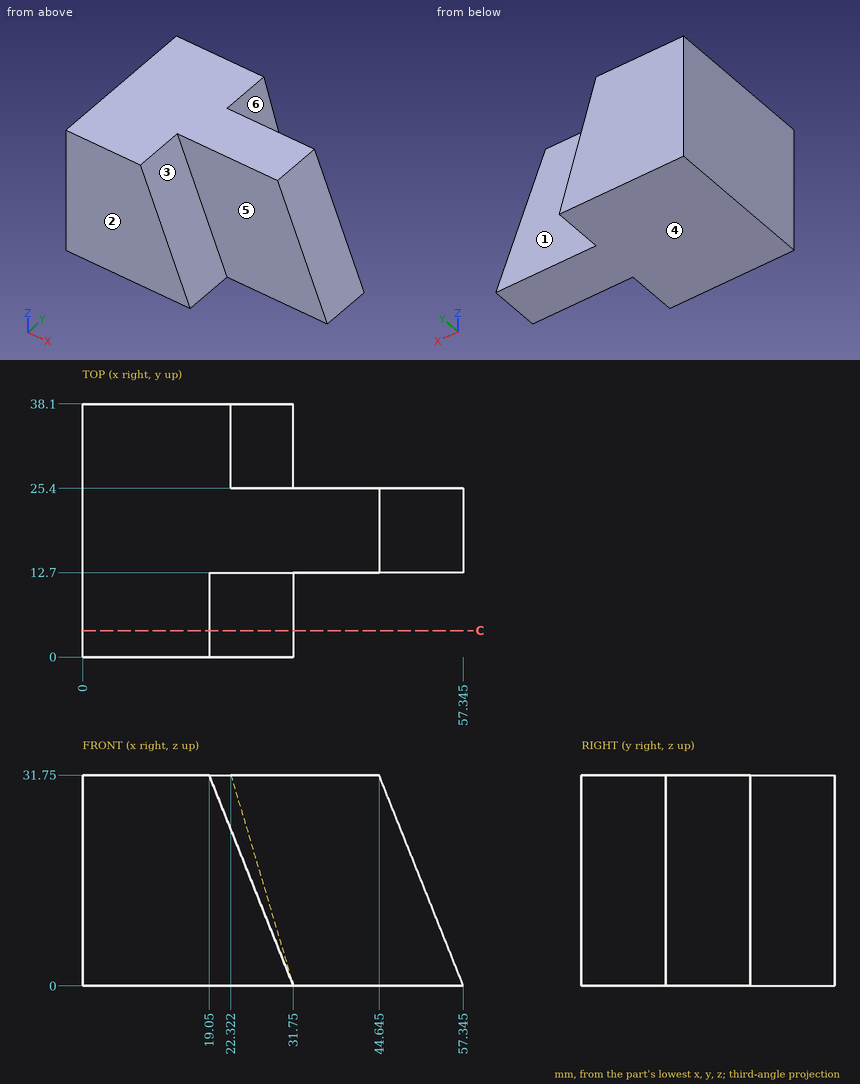
Design review of the part shown in the three views and the two pictorial views. Dimensions are in mm from the part's minimum x, y and z. A direction names the side the tool comes from. Give positions to 0.01 mm unless a question says otherwise; leave off trailing zeros. Order: outer loops, then holes, each group sorted by start corner. A loop starts at its lowest first (then second) coordinate and runs counter-clockwise, first axis right, second up. Notation, with made-up numbers: (-7, -33.75) -> (0, -33.75) arc R28 cw to (0, -11.75) -> close; hole circle Ø9 at (11.5, -15.5). An arc over 180 degrees is marked (long way). Write each question's results on one line, items separated by ' | '. Start each with the question number.
Q1. Machinability: for the marked faces 1, 2 and 3, which of the approach directions +Z, -Z, +X, -X, +Y, -Y give a long, thin tool a straight path to every point of the face, cutting with its end or side? Answer none if there is none.
Q2. Add section C-C on y = 4. Give the boundary of the cut face in (x, z).
Q3. Mouldability with a two-part tool opening along Z and no side actions: class the marked faces 4, 5 and 6 as +Z half, -Z half, draft (parallel to the pull), parting line (faces both ways), or undercut.
Q4. For pin 1 (4 mm diameter, centred on y = 13, z = 14.5, fed in from +X) (1 decimal); pin 2 (10 mm diameter, centred on y = 16, z = 27, fed in from +X) (1 decimal); pin 3 (5 mm diameter, centred on x = 51.5, z = 16.5, fed in from -Y), all flat-tipped, find the tip position at first contact; note any pin that passes through.
Q5. Wall thickness on L1, parallel to Y at x = 36, z = 19.5; L2, parallel to Y at x = 29, z = 8.5; L3, parallel to X at y = 26, z = 12: over which ranges is each line inside the solid? List them lowest first. Write a range as from..to.
Found:
1) face 1: +Z, +X, +Y | face 2: +Z, -Z, +X, -X, -Y | face 3: +Z, +X, -Y
2) outline: (0, 0) -> (31.75, 0) -> (19.05, 31.75) -> (0, 31.75) -> close
3) face 4: -Z half | face 5: draft | face 6: +Z half
4) pin 1: stops at x = 52.3 | pin 2: stops at x = 48.5 | pin 3: stops at y = 12.7
5) L1: y = 12.7..25.4 | L2: y = 12.7..38.1 | L3: x = 0..28.19
